CAD build for the part. Positions are in the model's coordinates, mm. A direction names the side the tool comes from. Round coordinates to 2 decimals unless told otherwise and drop trailing zeros. Loops run counter-clockwise (first coordinate to the right, second up) from the corner with the lowest first, then second, coordinate; pieces in that order, holes last. Notation, with made-up numbers: (61, 76) -> (97, 76) arc R26 ccw to (97, 94) -> close; hole circle Ø2 at (60, 20.5). An arc over 180 degrees is marked (long way). Answer as CSV lines item,"result".
```python
from build123d import *

# Parameters (mm, degrees)
BOSS_EXTRUDE1_DEPTH = 4
SKETCH5_R           = 4.7625
CUT_EXTRUDE1_DEPTH  = 272.785715814
SKETCH8_R           = 3.175
CUT_EXTRUDE3_DEPTH  = 272.785715814


with BuildPart() as part:
    # Sketch1 → Boss-Extrude1 (new body)
    with BuildSketch(Plane(origin=(0, 0, 0), x_dir=(1, 0, 0), z_dir=(0, 1, 0))):
        with BuildLine():
            Line((-55.078065391, 65.670374736), (-15.882456002, -41.901827969))
            ThreePointArc((-15.882456002, -41.901827969), (-15.529329867, -43.032283758), (-15.283044075, -44.190718765))
            Line((-15.283044075, -44.190718765), (12.6911511, -214.459876374))
            ThreePointArc((12.6911511, -214.459876374), (2.218090383, -229.050798182), (-12.372831425, -218.577737465))
            Line((-12.372831425, -218.577737465), (-36.044890736, -74.494178583))
            Line((-36.044890736, -74.494178583), (-123.815593368, -172.591431542))
            ThreePointArc((-123.815593368, -172.591431542), (-141.748449811, -173.587754678), (-142.744772948, -155.654898235))
            Line((-142.744772948, -155.654898235), (-42.351793784, -43.450310863))
            Line((-42.351793784, -43.450310863), (-78.943224061, 56.974732054))
            ThreePointArc((-78.943224061, 56.974732054), (-71.358466067, 73.25513273), (-55.078065391, 65.670374736))
        make_face()
    extrude(amount=BOSS_EXTRUDE1_DEPTH)

    # Sketch5 → Cut-Extrude1 (cut, through all)
    with BuildSketch(Plane(origin=(0, 4, 0), x_dir=(1, 0, 0), z_dir=(0, 1, 0))):
        with Locations(Location((-27.815035337, -46.24964931, 0), (0, 0, 270))):
            Circle(SKETCH5_R)
    extrude(amount=-CUT_EXTRUDE1_DEPTH, mode=Mode.SUBTRACT)

    # Sketch8 → Cut-Extrude3 (cut, through all)
    with BuildSketch(Plane(origin=(0, 4, 0), x_dir=(1, 0, 0), z_dir=(0, 1, 0))):
        with Locations(Location((-67.010644726, 61.322553395, 0), (0, 0, 270))):
            Circle(SKETCH8_R)
        with Locations(Location((0.159159837, -216.518806919, 0), (0, 0, 270))):
            Circle(SKETCH8_R)
        with Locations(Location((-133.280183158, -164.123164888, 0), (0, 0, 270))):
            Circle(SKETCH8_R)
    extrude(amount=-CUT_EXTRUDE3_DEPTH, mode=Mode.SUBTRACT)


solid = part.part
```
Q1. Slice it at B-B, the plane z = -33.5. Give the cut face in (x, y), and give its area (3 significant figures).
Results:
outline,"(-70.39, 0) -> (-43.36, 0) -> (-43.36, 4) -> (-70.39, 4) -> close"
area,"108 mm2"
Q2. Two-plate mould, pull along X, no slides. Class faces 4 (the flat face through (-49, 4, 88)), 5 (the cylindrical face through (-72, 2, -73)), 6 (the cylindrical face through (-63.863, 2.028, -61.736)), 7 (the cylindrical face through (-141.54, 1.97, 173.77)): pulls with the +X half, pulls with the -X half, needs draft (parallel to the pull), parting line crosses it, or undercut.
Results:
face 4,"needs draft"
face 5,"parting line crosses it"
face 6,"undercut"
face 7,"undercut"
Q3. Drop flat-ended pins along their axis: pin 1 Ø2 at (x, y) = (-56.5, 0.5) entering from -Z; pin 2 Ø8.5 at (x, z) = (-133.28, 164.12) entering from +Y; pin 3 Ø1.5 at (x, y) = (-87.5, 1.5) entering from +Z. Give the stop position or say it passes through.
Results:
pin 1,"z = -69.74"
pin 2,"y = 4"
pin 3,"z = 132.84"
Q4. Tool access for faces 1 (the flat face through (-24.043, 1.972, 147.545)), 2 (the flat face through (-1.492, 1.972, 128.133)), 3 (the flat face through (-60.39, 1.97, -6.06)): list every direction of +Z, -Z, +X, -X, +Y, -Y with a clear straight run to the whole face (end or side of a thin tool).
Results:
face 1,"+Z, +Y, -Y"
face 2,"-Z, +X, +Y, -Y"
face 3,"-X, +Y, -Y"
Q5. Slice it at A-A, the plane y = 1.95. Count the separate pieces of the cut face and the enclosed holes in it, and give its area (3 significant figures).
Results:
separate pieces,"1"
enclosed holes,"4"
area,"11,500 mm2"
Q6. Probe L1, parallel to X at y = 0.8, z = 214; L2, parallel to X at y = 3.05, z = 150.5; L3, parallel to X at y = 3.55, z = 166.5. List the from-to ranges inside material, lowest first. Write a range as [from, to].
Results:
L1,"[-13.12, -1.77], [2.09, 12.62]"
L2,"[-138.13, -104.05], [-23.56, 2.18]"
L3,"[-145.76, -135.39], [-131.18, -118.37], [-20.93, 4.81]"
Q7. Slice it at C-C, the plane x = -87. Give the cut face in (y, z).
Results:
outline,"(0, 93.35) -> (4, 93.35) -> (4, 131.44) -> (0, 131.44) -> close"
